Geometry: final body of the model. Coordinates: model frame, mm. Coordinates: 2 decimals unless noted, no trailing zeros. Order: outer loops, then holes, each group sorted by start corner. A loop starts at its lowest first (then second) coordinate and runs counter-clockwise, first axis right, second up. Notation, with made-up numbers: M 3,35.5 L 61,35.5 A24 cw 61,64.5 Z; hole C 15,34 d1. An arc over 180 degrees is marked long. One line per question, with ' | ' between items.
from build123d import *

# Parameters (mm, degrees)
SKETCH_1_W               = 25
SKETCH_1_H               = 116
EXTRUDE_1_DEPTH          = 4
SKETCH_2_R               = 1.525
CUT_EXTRUDE_1_DEPTH      = 1
CUT_EXTRUDE_1_DEPTH_BACK = 5
FILLET_1_R               = 3
CUT_EXTRUDE_2_DEPTH      = 1
CUT_EXTRUDE_2_DEPTH_BACK = 5


with BuildPart() as part:
    # 草图1 → 凸台-拉伸1 (new body)
    with BuildSketch(Plane.XY):
        Rectangle(SKETCH_1_W, SKETCH_1_H)
    extrude(amount=EXTRUDE_1_DEPTH)

    # 草图2 → 切除-拉伸1 (cut, two sides)
    with BuildSketch(Plane(origin=(0, 0, 0), x_dir=(-1, 0, 0), z_dir=(0, 0, -1))) as cut_extrude_1_sk:
        with Locations((0, -54.000000001)):
            Circle(SKETCH_2_R)
        with Locations((0, -24.000000001)):
            Circle(SKETCH_2_R)
        with Locations((0, 5.999999999)):
            Circle(SKETCH_2_R)
        with Locations((0, 35.999999999)):
            Circle(SKETCH_2_R)
    extrude(amount=CUT_EXTRUDE_1_DEPTH, mode=Mode.SUBTRACT)
    extrude(cut_extrude_1_sk.sketch, amount=-CUT_EXTRUDE_1_DEPTH_BACK, mode=Mode.SUBTRACT)

    # 圆角1
    fillet_1_edges = [part.edges().sort_by_distance(p)[0] for p in [
        (12.5, -58, 2),
        (-12.5, -58, 2),
        (-12.5, 58, 2),
        (12.5, 58, 2),
    ]]
    fillet(fillet_1_edges, radius=FILLET_1_R)

    # 草图4 → 切除-拉伸2 (cut, two sides)
    with BuildSketch(Plane.XY.offset(4)) as cut_extrude_2_sk:
        with BuildLine():
            Line((-5, 14.999999999), (-5, 26.999999999))
            ThreePointArc((-5, 26.999999999), (0, 31.999999999), (5, 26.999999999))
            Line((5, 26.999999999), (5, 14.999999999))
            ThreePointArc((5, 14.999999999), (0, 9.999999999), (-5, 14.999999999))
        make_face()
        with BuildLine():
            Line((-5, -45.000000001), (-5, -33.000000001))
            ThreePointArc((-5, -33.000000001), (0, -28.000000001), (5, -33.000000001))
            Line((5, -33.000000001), (5, -45.000000001))
            ThreePointArc((5, -45.000000001), (0, -50.000000001), (-5, -45.000000001))
        make_face()
        with BuildLine():
            Line((-5, -15.000000001), (-5, -3.000000001))
            ThreePointArc((-5, -3.000000001), (0, 1.999999999), (5, -3.000000001))
            Line((5, -3.000000001), (5, -15.000000001))
            ThreePointArc((5, -15.000000001), (0, -20.000000001), (-5, -15.000000001))
        make_face()
        with BuildLine():
            Line((-5, 44.499999999), (-5, 49.499999999))
            ThreePointArc((-5, 49.499999999), (0, 54.499999999), (5, 49.499999999))
            Line((5, 49.499999999), (5, 44.499999999))
            ThreePointArc((5, 44.499999999), (0, 39.499999999), (-5, 44.499999999))
        make_face()
    extrude(amount=CUT_EXTRUDE_2_DEPTH, mode=Mode.SUBTRACT)
    extrude(cut_extrude_2_sk.sketch, amount=-CUT_EXTRUDE_2_DEPTH_BACK, mode=Mode.SUBTRACT)


solid = part.part
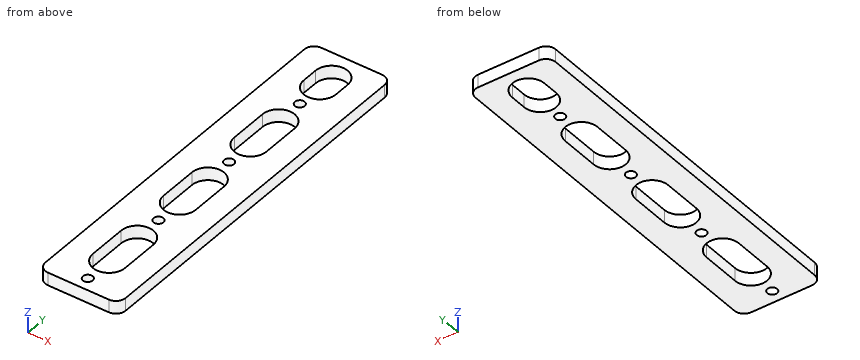
1. Material intervals for line 1 (X direction, y = 36, z = 2.8) (3 decimals); line 2 (X direction, y = -12, z = 1.95); line 3 (Y direction, x = 11, z = 1.3), sorted ascending. Write a range as [from, to].
Response values:
line 1: x = [-12.5, -1.525], [1.525, 12.5] | line 2: x = [-12.5, -5], [5, 12.5] | line 3: y = [-57.6, 57.6]
2. Pin query (flat end, axial travel): P1, Ø2.5, axis at x = 0, y = 6, coming from the +Z side. Return the tip coordinate at first contact, or that it passes through.
Response values:
P1: passes through
3. Section B-B, the plane z = 2.3. Give the number of separate pieces and of enclosed holes in the cut face, and give its area (3 significant figures).
Response values:
separate pieces: 1 | enclosed holes: 8 | area: 2,140 mm^2
4. Section C-C, the plane y = 41.5. Output: boundary loops of the cut face in (x, z).
Response values:
outline: M -12.5,0 L -4,0 L -4,4 L -12.5,4 Z; M 4,0 L 12.5,0 L 12.5,4 L 4,4 Z
5. Section A-A, the plane y = 6. Output: boundary loops of the cut face in (x, z) (3 decimals).
Response values:
outline: M -12.5,0 L -1.525,0 L -1.525,4 L -12.5,4 Z; M 1.525,0 L 12.5,0 L 12.5,4 L 1.525,4 Z
